```python
from build123d import *

# Parameters (mm, degrees)
ESQUISSE1_R                  = 8
ESQUISSE1_R_2                = 4
BOSS_EXTRU_1_DEPTH           = 3
ESQUISSE1_4_R                = 4
BOSS_EXTRU_3_DEPTH           = 31.5
ENL_V_MAT_EXTRU_1_DEPTH      = 10
ENL_V_MAT_EXTRU_1_DEPTH_BACK = 10
ESQUISSE2_R                  = 1.6


with BuildPart() as part:
    # Esquisse1 → Boss.-Extru.1 (new body)
    with BuildSketch(Plane(origin=(0, 0, 0), x_dir=(1, 0, 0), z_dir=(0, 1, 0))):
        with Locations(Location((0, 0, 0), (0, 0, 270))):
            Circle(ESQUISSE1_R)
        with Locations(Location((0, 0, 0), (0, 0, 270))):
            Circle(ESQUISSE1_R_2, mode=Mode.SUBTRACT)
    extrude(amount=BOSS_EXTRU_1_DEPTH)

    # Esquisse1_4 → Boss.-Extru.3 (add)
    with BuildSketch(Plane(origin=(0, 0, 0), x_dir=(1, 0, 0), z_dir=(0, 1, 0))):
        with Locations(Location((0, 0, 0), (0, 0, 270))):
            Circle(ESQUISSE1_4_R)
    extrude(amount=BOSS_EXTRU_3_DEPTH)

    # Esquisse2 → Enl_v. mat.-Extru.1 (cut, two sides: drawn at the far end of the back side and taken through both)
    with BuildSketch(Plane.XY.offset(-ENL_V_MAT_EXTRU_1_DEPTH_BACK)):
        with Locations(Location((0, 26, 0), (0, 0, 90.000000001))):
            Circle(ESQUISSE2_R)
    extrude(amount=ENL_V_MAT_EXTRU_1_DEPTH + ENL_V_MAT_EXTRU_1_DEPTH_BACK, mode=Mode.SUBTRACT)


solid = part.part
```
CAD build for the part. Positions are in the model's coordinates, mm. Round coordinates to 2 decimals unless told otherwise and drop trailing zeros. Order: outer loops, then holes, each group sorted by start corner. A loop starts at its lowest first (then second) coordinate and runs counter-clockwise, first axis right, second up. Notation, with made-up numbers: (-3.75, -28) - (4.25, -28) arc R28 ccw to (4.25, -9) - close; hole circle Ø2 at (-16, 10). An arc over 180 degrees is marked (long way). Use CSV: the item, a comma, the result in double quotes. Start each with the question number.
1) Saw through at D-D (y = 22). List the corners of the cut face in (x, z), and give its area (3 significant figures).
2) Saw through at A-A (x = 0). List the corners of the cut face in (y, z), and give its area (3 significant figures).
3) Wall check: L1, parallel to Y at x = 0, z = 0; L2, parallel to Y at x = -5.5, z = -4.25; L3, parallel to X at y = 26, z = 2.75. Give the ranges that are in metal, low to high. Write a range as [from, to].
4) Saw through at B-B (z = 0). List the corners of the cut face in (x, y).
5) Saw through at C-C (x = 3). List the corners of the cut face in (y, z), and give its area (3 significant figures).
6) Two-plate mould, pull along X, no slides. Class faces 1 (the cylindrical face through (-0.481, 27.526, -0.058)), 2 (the flat face through (-2, 3, -4)), 3 (the cylindrical face through (-3.905, 17.05, -0.867)): pulls with the +X half, pulls with the -X half, needs draft (parallel to the pull), parting line crosses it, or undercut.
7) Pin check, flat tips, straight feed: pin 1 Ø3 at (x, y) = (0, 8.5) entering from -Z; pin 2 Ø6 at (y, z) = (6.5, -1.5) entering from -X; pin 3 Ø4 at (x, y) = (0, 26) entering from +Z; pin 4 Ø6 at (x, z) = (-4, -5.5) entering from -Y. Stop position of each tip, or through.
Values follow:
1,outline,"circle Ø8 at (0, 0)"
1,area,"50.3 mm2"
2,outline,"(0, -8) - (3, -8) - (3, -4) - (24.4, -4) - (24.4, 4) - (3, 4) - (3, 8) - (0, 8) - close; (27.6, -4) - (31.5, -4) - (31.5, 4) - (27.6, 4) - close"
2,area,"250 mm2"
3,L1,"y = [0, 24.4], [27.6, 31.5]"
3,L2,"y = [0, 3]"
3,L3,"x = [-2.9, -1.6], [1.6, 2.9]"
4,outline,"(-8, 0) - (8, 0) - (8, 3) - (4, 3) - (4, 31.5) - (-4, 31.5) - (-4, 3) - (-8, 3) - close; hole circle Ø3.2 at (0, 26)"
5,outline,"(0, -7.42) - (3, -7.42) - (3, -2.65) - (31.5, -2.65) - (31.5, 2.65) - (3, 2.65) - (3, 7.42) - (0, 7.42) - close"
5,area,"195 mm2"
6,face 1,"undercut"
6,face 2,"needs draft"
6,face 3,"parting line crosses it"
7,pin 1,"stops at z = -4"
7,pin 2,"stops at x = -4"
7,pin 3,"stops at z = 4"
7,pin 4,"stops at y = 0"
